Autodesk Inventor part; units mm, degrees
ref_plane "YZ Plane" through (0, 0, 0) normal (1, 0, 0) x (0, 1, 0)
ref_plane "XZ Plane" through (0, 0, 0) normal (0, 1, 0) x (-1, 0, 0)
ref_plane "XY Plane" through (0, 0, 0) normal (0, 0, 1) x (1, 0, 0)
sketch "Sketch1" plane through (0, 0, 0) normal (0, 1, 0) x (-1, 0, 0)
  line L0 (0, 0) -> (-80, 0)
  line L1 (-80, 0) -> (-80, -5)
  line L2 (-80, -5) -> (0, -5)
  line L3 (0, -5) -> (0, 0)
  dimension "d0" = 80
  dimension "d1" = 5
extrude "Extrusion1" add sketch "Sketch1" along normal blind 100
sketch "Sketch2" plane through (0, 100, 0) normal (0, 1, 0) x (1, 0, 0)
  line L0 (0, 0) -> (10, 0)
  line L1 (10, 0) -> (10, 2.5)
  line L2 (10, 2.5) -> (0, 2.5)
  line L3 (0, 2.5) -> (0, 0)
  circle A0 centre (10, 2.5) radius 1.75
  dimension "d4" = 10
  dimension "d5" = 2.5
  dimension "d6" = 3.5
extrude "Extrusion2" add sketch "Sketch2" along normal blind 5 contours A0 L2 L1 | L1 L2 A0
sketch "Sketch3" plane through (0, 100, 0) normal (0, 1, 0) x (1, 0, 0)
  line L0 (80, 5) -> (0, 5)
  line L1 (80, 5) -> (70, 5)
  line L2 (70, 5) -> (70, 2.5)
  line L3 (70, 2.5) -> (80, 2.5)
  line L4 (80, 2.5) -> (80, 5)
  circle A0 centre (70, 2.5) radius 1.75
  point P0 (0, 0)
  dimension "d9" = 10
  dimension "d10" = 2.5
  dimension "d11" = 3.5
extrude "Extrusion3" add sketch "Sketch3" along normal blind 5 contours A0 L3 L2 | L2 L3 A0
sketch "Sketch4" plane through (0, 0, 0) normal (0, 0, 1) x (1, 0, 0)
  line L0 (0, 0) -> (80, 0)
  line L1 (80, 0) -> (40, 0)
  line L2 (40, 0) -> (40, 80)
  line L3 (40, 80) -> (80, 80)
  line L4 (80, 80) -> (80, 0)
  line L5 (40, 80) -> (30, 80)
  line L6 (30, 80) -> (30, 85)
  line L7 (30, 85) -> (40, 85)
  line L8 (40, 85) -> (40, 80)
  dimension "d14" = 40
  dimension "d15" = 80
  dimension "d16" = 10
  dimension "d17" = 5
extrude "Extrusion4" cut sketch "Sketch4" against normal blind 10 contours L5 L6 L7 L8
properties part number "expo4"
Geometry: final body of the model. Coordinates: model frame, mm. A direction names the side the tool comes from. Round coordinates to 2 decimals unless told otherwise and drop trailing zeros. Order: outer loops, then holes, each group sorted by start corner. A loop starts at its lowest first (then second) coordinate and runs counter-clockwise, first axis right, second up. Notation, with made-up numbers: (5, 51.25) -> (46, 51.25) arc R16 ccw to (46, 82.25) -> close; hole circle Ø9 at (-30, 45). An arc over 180 degrees is marked (long way). Use one line per item in the form item = value.
(1) Section A-A on z = -3.3. Return loops of the section in (x, y), and give its area (3 significant figures).
Results list:
outline = (0, 0) -> (80, 0) -> (80, 100) -> (71.56, 100) -> (71.56, 105) -> (68.44, 105) -> (68.44, 100) -> (11.56, 100) -> (11.56, 105) -> (8.44, 105) -> (8.44, 100) -> (0, 100) -> close; hole (30, 80) -> (40, 80) -> (40, 85) -> (30, 85) -> close
area = 7,980 mm^2
(2) Section B-B on x = 41.5. Return loops of the section in (y, z), and give its area (3 significant figures).
Results list:
outline = (0, -5) -> (100, -5) -> (100, 0) -> (0, 0) -> close
area = 500 mm^2
(3) Access query for faces 4 (the face through (30, 82, -2)), 5 (the face through (71.669, 102.465, -1.974)), 6 (the face through (39, 49, 0)). Directions: +Z, -Z, +X, -X, +Y, -Y. A direction counts if a zero-diameter tool reaches every point of the face in a straight line with its end or side. Return the directions, or none.
Results list:
face_4 = +Z, -Z
face_5 = +Y
face_6 = +Z, +X, -X, +Y, -Y
(4) Draft query along Y for faces 1 (the face through (35, 85, -2)), 2 (the face through (41, 0, -2)), 3 (the face through (11.617, 102.465, -3.17)). Return one class per face: pulls with the +Y half, pulls with the -Y half, needs draft (parallel to the pull), parting line crosses it, or undercut.
Results list:
face_1 = undercut
face_2 = pulls with the -Y half
face_3 = needs draft
(5) Ray query, probe 1 along Y at (x, z) = (39, -1.8); probe 2 along Y at (x, z) = (11.5, -0.7). Return the intervals inside material, ascending. Write a range as [from, to].
Results list:
probe_1 = [0, 80], [85, 100]
probe_2 = [0, 100]
